Read the model definition and answer for the solid it produces. Units are mm, in the model's axes. A direction names the side the tool comes from. Give positions to 0.01 mm unless a question says otherwise; leave off trailing zeros. Loops run counter-clockwise (first coordinate to the right, second up) from the corner with the lowest first, then second, coordinate; pieces in that order, holes last. Notation, with made-up numbers: (5, 70) - (64, 70) arc R12 ccw to (64, 89) - close; hole circle Ø3 at (67, 47). An arc over 180 degrees is marked (long way). Write each question's results on one line, items separated by ' | '. Start each with the question number.
Q1. The part is cut by section C-C, the plane y = 75. Write down the section's boundary in (x, z).
Q2. The part is cut by section D-D, the plane y = -8. Write down the section's boundary in (x, z), plus the area to 3 significant figures.
Q3. For faces 1 (the flat face through (61.36, -21.51, 1.97)), 2 (the flat face through (48.8, -26.4, 2)), determine the directions among +Z, -Z, +X, -X, +Y, -Y from which every point of the face is accessible in a straight line to the end or side of a thin tool.
Q4. Determine the mould class of faces 3 (the cylindrical face through (12.04, 58.47, 1.97)), 4 (the cylindrical face through (92.924, -54.177, 1.972)), 5 (the flat face through (40.59, -34.84, 1.97)), 6 (the flat face through (29, -8, 0)) for opening direction Y: +Y half, -Y half, draft (parallel to the pull), parting line (faces both ways), or undercut.
Q5. Given pin 1 (1.5 mm diameter, centred on y = 17.5, z = 2.5, fed in from +X); pin 2 (1.2 mm diameter, centred on y = 92, z = 1.5, fed in from +X); pin 3 (2 mm diameter, centred on y = -62, z = 2.5, fed in from -X); pin 4 (8.5 mm diameter, centred on x = 70.95, y = -77.51, fed in from -Z), each flat-ended and moving along its own axis, determine where each tip first touches the part or whether it passes through.
Q6. The part is cut by section A-A, the plane y = 25. Write down the section's boundary in (x, z).
Q7. Find the intervals of material crossed by line 1 (X direction, y = 78, z = 3.1); line 2 (Y direction, x = 71.5, z = 2.85); line 3 (Y direction, x = 30, z = 0.75), in increasing order. Write a range as from..to.
Q8. The part is cut by section B-B, the plane z = 2.9. State how many separate pieces and enclosed holes the cut face has, plus the area to 3 significant figures.
```python
from build123d import *

# Parameters (mm, degrees)
SKETCH1_R           = 3.5
SKETCH1_R_2         = 7
SKETCH1_R_3         = 4
BOSS_EXTRUDE1_DEPTH = 4


with BuildPart() as part:
    # Sketch1 → Boss-Extrude1 (new body)
    with BuildSketch(Plane.XY):
        with BuildLine():
            Line((55.379885617, -96.237749993), (83.664156864, -96.237749993))
            ThreePointArc((83.664156864, -96.237749993), (90.735224676, -93.308817805), (93.664156864, -86.237749993))
            Line((93.664156864, -86.237749993), (93.664156864, -57.953478746))
            ThreePointArc((93.664156864, -57.953478746), (92.902952189, -54.126644422), (90.735224676, -50.882410934))
            Line((90.735224676, -50.882410934), (31.159701747, 8.693111995))
            ThreePointArc((31.159701747, 8.693111995), (26.824246721, 15.181578972), (25.301837371, 22.835247619))
            Line((25.301837371, 22.835247619), (25.301837371, 125))
            ThreePointArc((25.301837371, 125), (23.837371277, 128.535533906), (20.301837371, 130))
            Line((20.301837371, 130), (5, 130))
            ThreePointArc((5, 130), (1.464466094, 128.535533906), (0, 125))
            Line((0, 125), (0, 5))
            Line((0, 5), (0, -36.715728753))
            ThreePointArc((0, -36.715728753), (1.52240935, -44.3693974), (5.857864376, -50.857864376))
            Line((5.857864376, -50.857864376), (48.308817805, -93.308817805))
            ThreePointArc((48.308817805, -93.308817805), (51.553051293, -95.476545318), (55.379885617, -96.237749993))
        make_face()
        with Locations((12.5, 55)):
            Circle(SKETCH1_R, mode=Mode.SUBTRACT)
        with Locations((12.5, 40)):
            Circle(SKETCH1_R, mode=Mode.SUBTRACT)
        with Locations((12.5, 25)):
            Circle(SKETCH1_R, mode=Mode.SUBTRACT)
        with Locations((70.953796111, -77.513095535)):
            Circle(SKETCH1_R_2, mode=Mode.SUBTRACT)
        with Locations((75.03834495, -45)):
            Circle(SKETCH1_R_3, mode=Mode.SUBTRACT)
        with BuildLine():
            Line((38.555717556, -15.716967459), (59.317673007, -37.372017813))
            ThreePointArc((59.317673007, -37.372017813), (59.142526441, -45.690498717), (50.824045538, -45.515352151))
            Line((50.824045538, -45.515352151), (30.062090086, -23.860301797))
            ThreePointArc((30.062090086, -23.860301797), (30.237236652, -15.541820893), (38.555717556, -15.716967459))
        make_face(mode=Mode.SUBTRACT)
        with BuildLine():
            ThreePointArc((8.5, 69), (12.5, 65), (16.5, 69))
            Line((16.5, 69), (16.5, 119))
            ThreePointArc((16.5, 119), (12.5, 123), (8.5, 119))
            Line((8.5, 119), (8.5, 69))
        make_face(mode=Mode.SUBTRACT)
        with BuildLine():
            ThreePointArc((36.446439435, -59.766764), (44.766764, -59.766764), (44.766764, -51.446439435))
            Line((44.766764, -51.446439435), (23.553560565, -30.233236))
            ThreePointArc((23.553560565, -30.233236), (15.233236, -30.233236), (15.233236, -38.553560565))
            Line((15.233236, -38.553560565), (36.446439435, -59.766764))
        make_face(mode=Mode.SUBTRACT)
    extrude(amount=BOSS_EXTRUDE1_DEPTH)


solid = part.part
```
Check sheet entries:
1) outline: (0, 0) - (8.5, 0) - (8.5, 4) - (0, 4) - close; (16.5, 0) - (25.3, 0) - (25.3, 4) - (16.5, 4) - close
2) outline: (0, 0) - (47.85, 0) - (47.85, 4) - (0, 4) - close | area: 191 mm^2
3) face 1: +Z, -Z, +X, +Y | face 2: +Z, -Z
4) face 3: undercut | face 4: +Y half | face 5: undercut | face 6: draft
5) pin 1: stops at x = 26.25 | pin 2: stops at x = 25.3 | pin 3: stops at x = 16 | pin 4: passes through
6) outline: (0, 0) - (9, 0) - (9, 4) - (0, 4) - close; (16, 0) - (25.3, 0) - (25.3, 4) - (16, 4) - close
7) line 1: x = 0..8.5, 16.5..25.3 | line 2: y = -96.24..-84.49, -70.53..-46.87, -43.13..-31.65 | line 3: y = -75..-53.32, -36.68..-23.79, -15.78..9.96
8) separate pieces: 1 | enclosed holes: 8 | area: 7,920 mm^2
